from build123d import *

# Parameters (mm, degrees)
SKETCH_R        = 25
PAD_DEPTH       = 4
POCKET_DEPTH    = 5
SKETCH009_W     = 8
SKETCH009_H     = 8
POCKET001_DEPTH = 5


with BuildPart() as part:
    # Sketch → Pad (new body)
    with BuildSketch(Plane.XY):
        Circle(SKETCH_R)
    extrude(amount=PAD_DEPTH)

    # Sketch008 → Pocket (cut)
    with BuildSketch(Plane(origin=(0, 0, 0), x_dir=(-1, 0, 0), z_dir=(0, 0, 1))):
        with BuildLine():
            add(Edge.make_bspline(
                [(10, 0), (10.72, 2.827433), (10.551736, 6.107253), (9.255372, 9.525547), (6.717902, 12.639095), (3.029145, 14.935747), (-1.475809, 15.944125), (-6.25069, 15.376552), (-10.669796, 13.21807), (-14.170604, 9.717764), (-16.358172, 5.315092)],
                knots=[0, 0, 0, 0, 0, 0, 0, 0, 0, 0, 0, 2.999063, 2.999063, 2.999063, 2.999063, 2.999063, 2.999063, 2.999063, 2.999063, 2.999063, 2.999063, 2.999063], degree=10))
            ThreePointArc((-16.358172, 5.315092), (-19.522596, 3.666166), (-21.113455, 6.860177))
            add(Edge.make_bspline(
                [(15, 0), (15.72, 4.24115), (15.107604, 8.934687), (12.922973, 13.609729), (9.116521, 17.666081), (3.904817, 20.464523), (-2.203607, 21.466288), (-8.476704, 20.39419), (-14.128959, 17.31496), (-18.489025, 12.607374), (-21.113455, 6.860177)],
                knots=[0, 0, 0, 0, 0, 0, 0, 0, 0, 0, 0, 2.999063, 2.999063, 2.999063, 2.999063, 2.999063, 2.999063, 2.999063, 2.999063, 2.999063, 2.999063, 2.999063], degree=10))
            ThreePointArc((15, 0), (12.5, -2.684775), (10, 0))
        make_face()
    extrude(amount=POCKET_DEPTH, mode=Mode.SUBTRACT)

    # Sketch009 → Pocket001 (cut)
    with BuildSketch(Plane.XY):
        with BuildLine():
            add(Edge.make_bspline(
                [(10, 0), (10.72, 2.827433), (10.551736, 6.107253), (9.255372, 9.525547), (6.717902, 12.639095), (3.029145, 14.935747), (-1.475809, 15.944125), (-6.25069, 15.376552), (-10.669796, 13.21807), (-14.170604, 9.717764), (-16.358172, 5.315092)],
                knots=[0, 0, 0, 0, 0, 0, 0, 0, 0, 0, 0, 2.999063, 2.999063, 2.999063, 2.999063, 2.999063, 2.999063, 2.999063, 2.999063, 2.999063, 2.999063, 2.999063], degree=10))
            ThreePointArc((-16.358172, 5.315092), (-19.522596, 3.666166), (-21.113455, 6.860177))
            add(Edge.make_bspline(
                [(15, 0), (15.72, 4.24115), (15.107604, 8.934687), (12.922973, 13.609729), (9.116521, 17.666081), (3.904817, 20.464523), (-2.203607, 21.466288), (-8.476704, 20.39419), (-14.128959, 17.31496), (-18.489025, 12.607374), (-21.113455, 6.860177)],
                knots=[0, 0, 0, 0, 0, 0, 0, 0, 0, 0, 0, 2.999063, 2.999063, 2.999063, 2.999063, 2.999063, 2.999063, 2.999063, 2.999063, 2.999063, 2.999063, 2.999063], degree=10))
            ThreePointArc((15, 0), (12.5, -2.684775), (10, 0))
        make_face()
        Rectangle(SKETCH009_W, SKETCH009_H)
    extrude(amount=POCKET001_DEPTH, mode=Mode.SUBTRACT)


solid = part.part
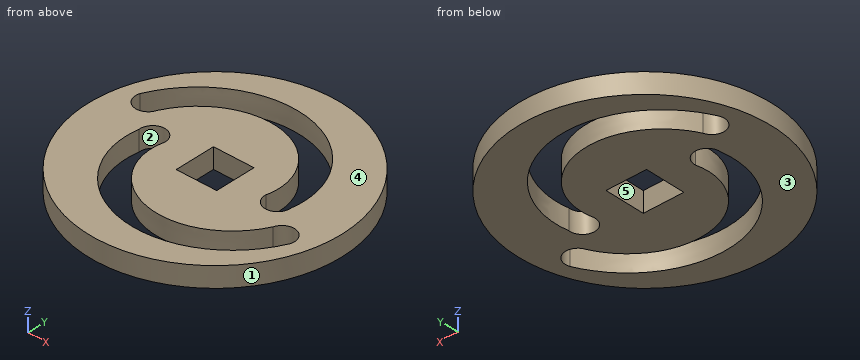
Geometry check sheet. Reference: the model listing, model coordinates, mm. Face numbers are marked on the shaded views. A direction names the side the tool comes from. Round coordinates to 2 decimals unless told otherwise and drop trailing zeros. One line per item, written item: value.
1. Scan lines: L1, parallel to X at y = 7, z = 1.6; L2, parallel to Y at x = 11.5, z = 2.1; L3, parallel to X at y = 6, z = 1.35. Record each from-to range of solid material in increasing order.
The answers:
L1: x = -24 to -21.05, -15.4 to 9.3, 14.55 to 24
L2: y = -22.2 to -16.99, -11.18 to -2.48, 12.69 to 22.2
L3: x = -24.27 to -21.25, -16 to 9.71, 14.81 to 24.27
2. Depth check by flat-ended pin: pin 1 Ø1 at (y, z) = (-17.5, 0.5) entering from -X; pin 2 Ø1.2 at (x, z) = (-2, 2.5) entering from +Y; pin 3 Ø1 at (y, z) = (-19.5, 1) entering from +X. Enter the tip coordinate at first touch or a pass-through.
The answers:
pin 1: stops at x = -18.33
pin 2: stops at y = 24.96
pin 3: stops at x = 16.25
3. Cross-section at A-A on x = 0. Give the number of separate pieces and of enclosed holes in the cut face, and give its area (3 significant figures).
The answers:
separate pieces: 4
enclosed holes: 0
area: 128 mm^2
4. Mould release check, pull along Y, two halves, no side actions. Record for the marked faces 1, 2 and 3: released by +Y, released by -Y, zero draft, split by the parting line, or undercut.
The answers:
face 1: split by the parting line
face 2: undercut
face 3: zero draft
5. Set-up check for the marked faces 4 and 5: record each of +Z, -Z, +X, -X, +Y, -Y from which the full face is reachable in a straight line by a thin tool's end or side.
The answers:
face 4: +Z, +X, -X, +Y, -Y
face 5: +Z, -Z
